The figure shows three views and two pictorial views of one solid part (mm, origin at its lowest corner). Answer the questions. A direction names the side the tool comes from. Coordinates: 2 decimals unless noted, no trailing zeros. Write each loop counter-clockwise with the first axis right and the second up, starting at its lowest first coordinate (ties: lowest second). Pieces come first, ordered by that corner, then holes.
Item 1: Section B-B (x = 10.5) is taken. Give the vertices of the cut face in (y, z).
Item 2: Section C-C (y = 12.5) is taken. Give the vertices of the cut face in (x, z).
Item 3: A tool of negligible diameter and unlimited length cuts with its end or side. For the marked faces 1, 2 and 3, from which of +Z, -Z, +X, -X, +Y, -Y can it reach the whole face along a straight path? Write none if from no direction.
Item 4: Straight lines are drawn through the part: probe 1 along Y at (x, z) = (3.5, 17); probe 2 along Z at (x, y) = (9.5, 8.5); probe 3 along X at (y, z) = (16, 14.5). For each, find the intervals that lie inside material, in ascending order.
Item 5: Section A-A (z = 9) is taken. Give the vertices of the cut face in (x, y), then the cut area to 3 significant figures.
Item 6: Section D-D (z = 5.25) is taken. Give the vertices of the cut face in (x, y), then the cut area to 3 significant figures.
Item 7: Each of these flat-tipped pins is pushed along its axis until it touches: P1, Ø10, axis at x = 7, y = 7.5, coming from the +Z side; P2, Ø4, axis at y = 12, z = 3, coming from the -X side; P3, Ø4.5, axis at x = 1.5, z = 5.5, coming from the -Y side; P4, Ø5, axis at x = 12, z = 2, coming from the -Y side. Where does it stop, or does it pass through?
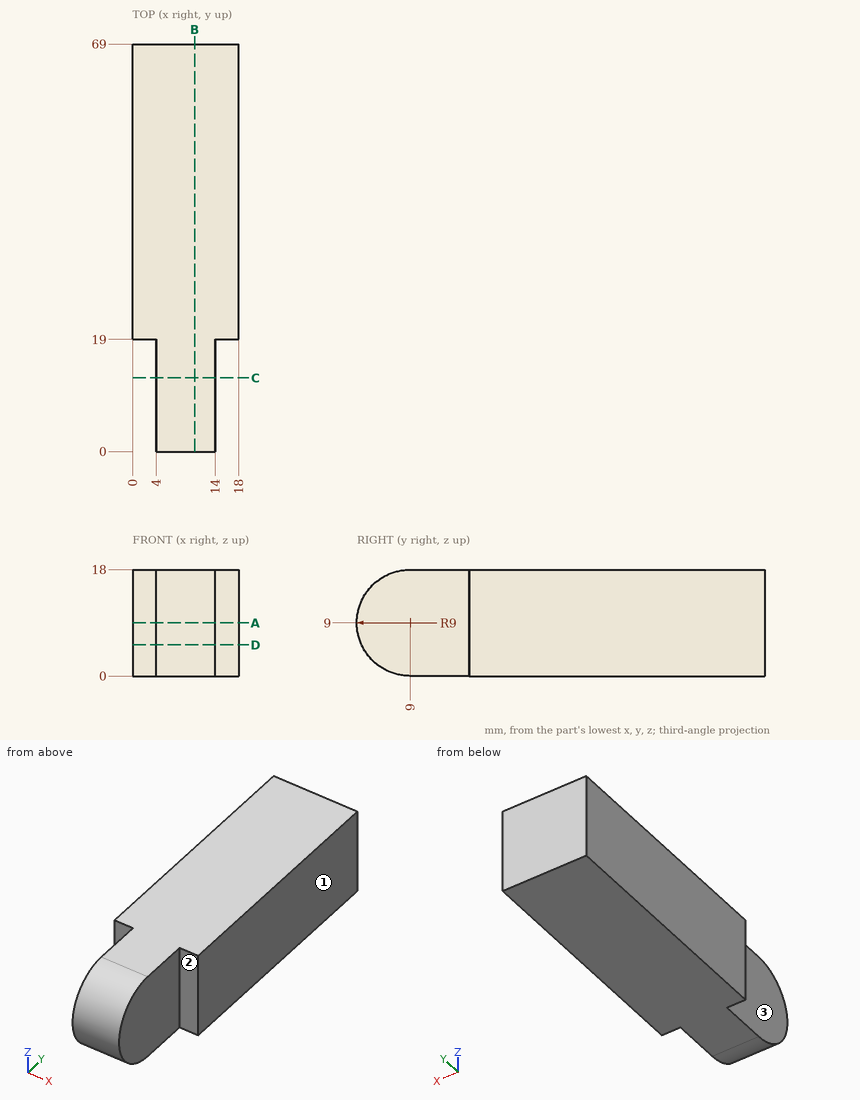
Established:
1. outline: (9, 0) - (69, 0) - (69, 18) - (9, 18) arc R9 ccw to start
2. outline: (4, 0) - (14, 0) - (14, 18) - (4, 18) - close
3. face 1: +Z, -Z, +X, +Y, -Y
3. face 2: +Z, -Z, +X, -Y
3. face 3: +Z, -Z, -X, -Y
4. probe 1: y = 19 to 69
4. probe 2: z = 0.01 to 17.99
4. probe 3: x = 4 to 14
5. outline: (0, 19) - (4, 19) - (4, 0) - (14, 0) - (14, 19) - (18, 19) - (18, 69) - (0, 69) - close
5. area: 1,090 mm2
6. outline: (0, 19) - (4, 19) - (4, 0.82) - (14, 0.82) - (14, 19) - (18, 19) - (18, 69) - (0, 69) - close
6. area: 1,080 mm2
7. P1: stops at z = 18
7. P2: stops at x = 4
7. P3: stops at y = 19
7. P4: stops at y = 1.21
